Geometry: see drawing. Coordinates: mm, zero at the bounding-box minimum. Round coordinates to 2 decimals unless told otherwise and drop trailing zeros. Order: outer loops, then holes, each group sorted by start corner. A loop starts at its lowest first (then second) coordinate and runs counter-clockwise, first axis right, second up. Notation, with made-up numbers: (51.5, 29.5) -> (68.5, 29.5) arc R6 cw to (68.5, 34.5) -> close; hole circle Ø5 at (89.5, -13). An arc over 180 degrees is marked (long way). Put each result on its own line as item: value.
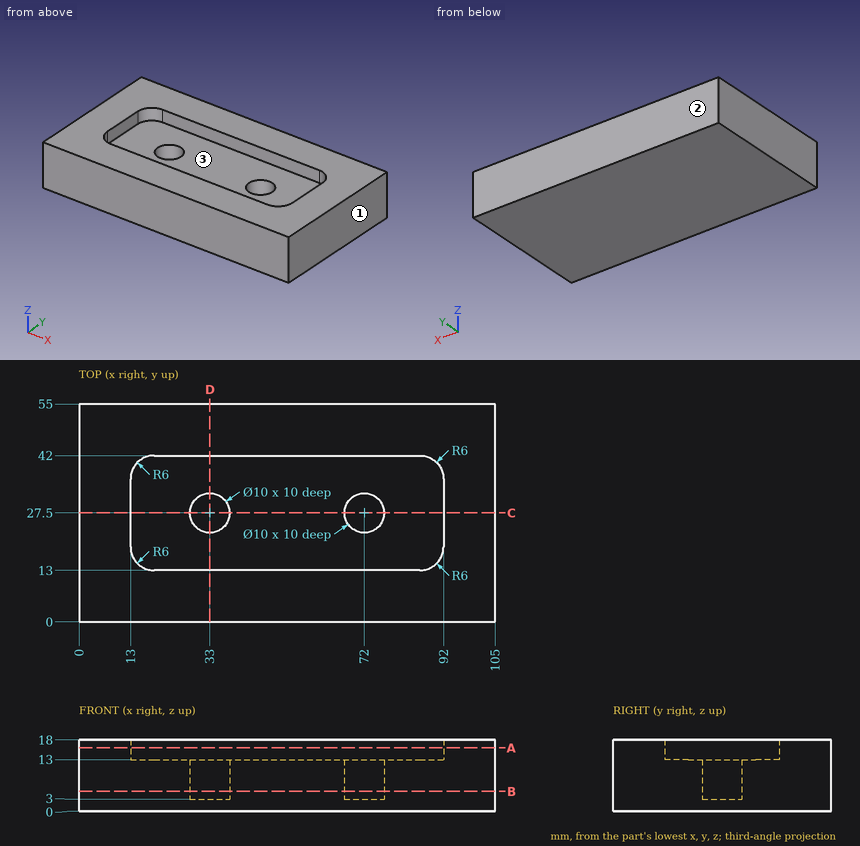
1. Cut plane B-B on z = 5. Return loops of the section in (x, y), and give its area (3 significant figures).
Ans:
outline: (0, 0) -> (105, 0) -> (105, 55) -> (0, 55) -> close; hole circle Ø10 at (33, 27.5); hole circle Ø10 at (72, 27.5)
area: 5,620 mm²
2. Cut plane A-A on z = 16. Return loops of the section in (x, y).
Ans:
outline: (0, 0) -> (105, 0) -> (105, 55) -> (0, 55) -> close; hole (13, 19) arc R6 ccw to (19, 13) -> (86, 13) arc R6 ccw to (92, 19) -> (92, 36) arc R6 ccw to (86, 42) -> (19, 42) arc R6 ccw to (13, 36) -> close
3. Material intervals for probe 1 along X at (y, z) = (27.5, 8); probe 2 along Y at (x, z) = (72, 8.5); probe 3 along X at (y, z) = (26.5, 14.75), sorted ascending.
Ans:
probe 1: 0 to 28, 38 to 67, 77 to 105
probe 2: 0 to 22.5, 32.5 to 55
probe 3: 0 to 13, 92 to 105
4. Cut plane C-C on y = 27.5. Return loops of the section in (x, z), and give its area (4 significant figures).
Ans:
outline: (0, 0) -> (105, 0) -> (105, 18) -> (92, 18) -> (92, 13) -> (77, 13) -> (77, 3) -> (67, 3) -> (67, 13) -> (38, 13) -> (38, 3) -> (28, 3) -> (28, 13) -> (13, 13) -> (13, 18) -> (0, 18) -> close
area: 1,295 mm²
5. Contact query for flat-ended pins moving along their axis: P1, Ø14.5, axis at x = 66, y = 25, coming from the +Z side; P2, Ø3, axis at x = 34.5, y = 27, coming from the +Z side. Output: stop coordinate, or through.
Ans:
P1: z = 13
P2: z = 3
6. Cut plane D-D on x = 33. Return loops of the section in (y, z), and give its area (3 significant figures).
Ans:
outline: (0, 0) -> (55, 0) -> (55, 18) -> (42, 18) -> (42, 13) -> (32.5, 13) -> (32.5, 3) -> (22.5, 3) -> (22.5, 13) -> (13, 13) -> (13, 18) -> (0, 18) -> close
area: 745 mm²
7. Draft query along Y for the marked faces 1, 2 and 3. Return one class per face: +Y half, -Y half, draft (parallel to the pull), parting line (faces both ways), or undercut.
Ans:
face 1: draft
face 2: +Y half
face 3: undercut
